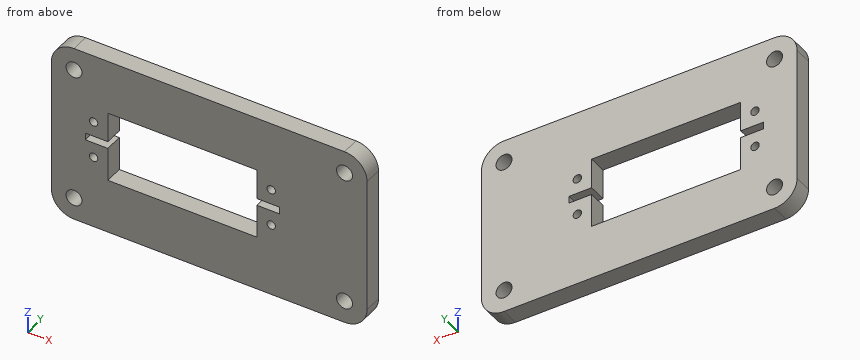
```python
from build123d import *

# Parameters (mm, degrees)
SKETCH1_W                       = 88.9
SKETCH1_H                       = 50.8
SKETCH1_W_2                     = 42.0000176
SKETCH1_H_2                     = 20
BOSS_EXTRUDE1_DEPTH             = 5.08
F_3_32_0_09375_DIAMETER_HOLE1_D = 2.38125
SKETCH4_W                       = 6.35
SKETCH4_H                       = 2
CUT_EXTRUDE1_DEPTH              = 6.08
FILLET2_R                       = 6.35
F_8_CLEARANCE_HOLE1_D           = 4.4958


with BuildPart() as part:
    # Sketch1 → Boss-Extrude1 (new body)
    with BuildSketch(Plane(origin=(0, 0, 0), x_dir=(1, 0, 0), z_dir=(0, 1, 0))):
        with Locations((-44.45, -25.4)):
            Rectangle(SKETCH1_W, SKETCH1_H)
        with Locations((-52.0249912, -25.4)):
            Rectangle(SKETCH1_W_2, SKETCH1_H_2, mode=Mode.SUBTRACT)
    extrude(amount=BOSS_EXTRUDE1_DEPTH)

    # 3/32 (0.09375) Diameter Hole1 (through all)
    with Locations(Plane(origin=(0, 5.08, 0), x_dir=(1, 0, 0), z_dir=(0, 1, 0))):
        with Locations((-77.0439912, -31.15), (-77.0439912, -20.65), (-27.0059912, -31.15), (-27.0059912, -20.65)):
            Hole(F_3_32_0_09375_DIAMETER_HOLE1_D / 2)

    # Sketch4 → Cut-Extrude1 (cut, through all)
    with BuildSketch(Plane(origin=(0, 5.08, 0), x_dir=(1, 0, 0), z_dir=(0, 1, 0))):
        with Locations((-76.2, -25.9)):
            Rectangle(SKETCH4_W, SKETCH4_H)
        with Locations((-27.8499824, -25.9)):
            Rectangle(SKETCH4_W, SKETCH4_H)
    extrude(amount=-CUT_EXTRUDE1_DEPTH, mode=Mode.SUBTRACT)

    # Fillet2
    fillet2_edges = [part.edges().sort_by_distance(p)[0] for p in [
        (-88.9, 2.54, 0),
        (0, 2.54, 0),
        (0, 2.54, 50.8),
        (-88.9, 2.54, 50.8),
    ]]
    fillet(fillet2_edges, radius=FILLET2_R)

    # #8 Clearance Hole1 (through all)
    with Locations(Plane(origin=(0, 5.08, 0), x_dir=(1, 0, 0), z_dir=(0, 1, 0))):
        with Locations((-82.55, -6.35), (-82.55, -44.45), (-6.35, -6.35), (-6.35, -44.45)):
            Hole(F_8_CLEARANCE_HOLE1_D / 2)


solid = part.part
```
Geometry check sheet. Reference: the model listing, model coordinates, mm. Give positions to 0.01 mm unless a question says otherwise; leave off trailing zeros. Write each loop counter-clockwise with the first axis right and the second up, starting at its lowest first coordinate (ties: lowest second). Pieces come first, ordered by that corner, then holes. Notation, with made-up numbers: (70, 82) - (84, 82) arc R6 ccw to (84, 88) - close; hole circle Ø7 at (-23.75, -34). An arc over 180 degrees is marked (long way). Use a Markdown table: item, result.
Q1. Section check C-C, the plane y = 4.25. Give the number of separate pieces and of enclosed holes in the cut face, then the cut area to 3 significant figures.
Computed:
| item | result |
|---|---|
| separate pieces | 1 |
| enclosed holes | 9 |
| area | 3,530 mm² |
Q2. Go/stop test with flat-tipped pins: P1, Ø7, axis at x = -82.55, z = 6.35, coming from the +Y side; P2, Ø1.4, axis at x = -27.01, z = 31.15, coming from the +Y side. Record where each tip stops, or that it passes through.
Computed:
| item | result |
|---|---|
| P1 | stops at y = 5.08 |
| P2 | passes through |
Q3. Section check A-A, the plane z = 18.5. Enter the section's corners in (x, y) (3 decimals).
Computed:
| item | result |
|---|---|
| outline | (-88.9, 0) - (-73.025, 0) - (-73.025, 5.08) - (-88.9, 5.08) - close; (-31.025, 0) - (0, 0) - (0, 5.08) - (-31.025, 5.08) - close |
Q4. Thickness scan on L1, parallel to X at y = 4.15, z = 44.5; L2, parallel to Z at x = -82.55, y = 3.6; L3, parallel to X at y = 2.9, z = 20.65 (3 decimals). Record the ranges inside material, lowest first. Write a range as [from, to].
Computed:
| item | result |
|---|---|
| L1 | x = [-88.9, -84.8], [-80.3, -8.6], [-4.1, 0] |
| L2 | z = [0, 4.1], [8.6, 42.2], [46.7, 50.8] |
| L3 | x = [-88.9, -78.235], [-75.853, -73.025], [-31.025, -28.197], [-25.815, 0] |
Q5. Section check B-B, the plane x = -62.5. Enter the section's corners in (y, z).
Computed:
| item | result |
|---|---|
| outline | (0, 0) - (5.08, 0) - (5.08, 15.4) - (0, 15.4) - close; (0, 35.4) - (5.08, 35.4) - (5.08, 50.8) - (0, 50.8) - close |
